Job drawing, mm, ordinate dimensions from the low corner. One solid piece. A direction names the side the tool comes from. Give positions to 0.01 mm unless a question says otherwise; leave off trailing zeros. Write each loop counter-clockwise with the first axis right and the second up, starting at its lowest first coordinate (ties: lowest second). Pieces come first, ordered by that corner, then holes. Notation, with made-up numbers: (36.25, 86) - (93.25, 86) arc R12 ccw to (93.25, 95) - close; hole circle Ø8 at (7.25, -2.75). An arc over 180 degrees is marked (long way). Answer as a JSON object with one key per item and string values.
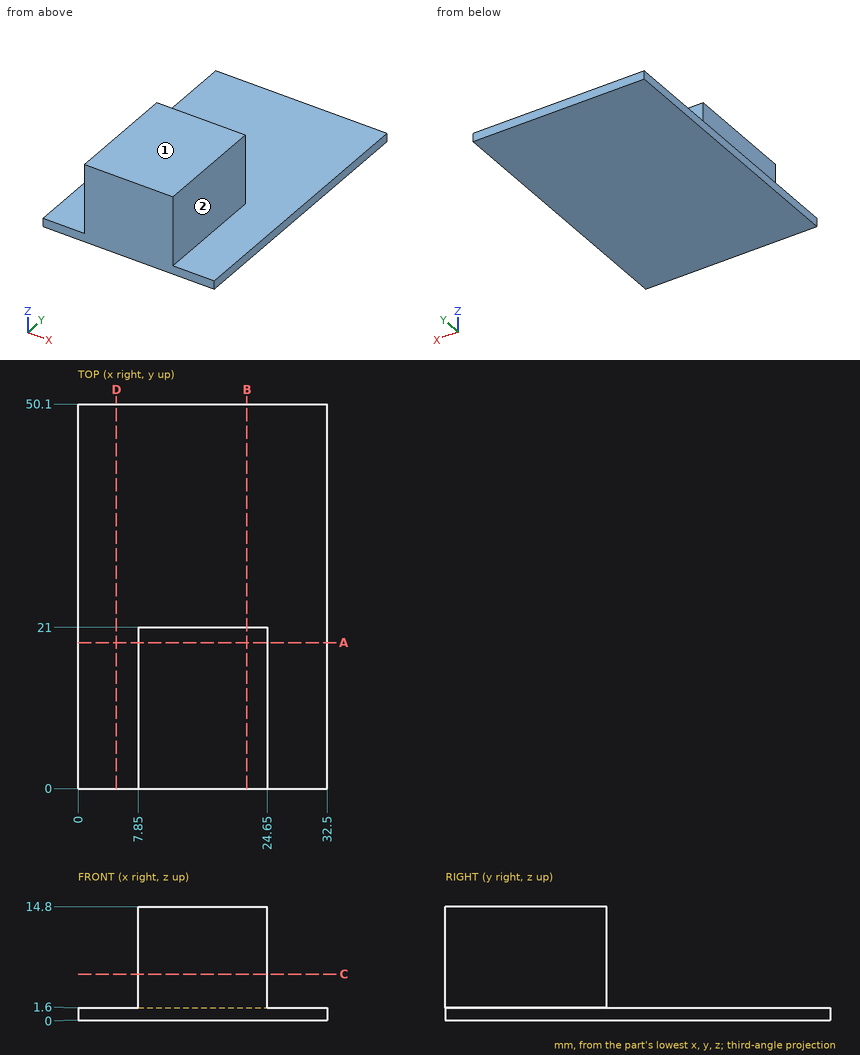
Item 1: Flat gauge pins, fed straight in: P1, Ø1.5, axis at x = 24, y = 30.5, coming from the +Z side; P2, Ø4, axis at x = 18.5, z = 6, coming from the +Y side; P3, Ø5, axis at y = 20.5, z = 13, coming from the -X side; P4, Ø1, axis at x = 26.5, y = 19, coming from the -Z side. Where does each tip first touch, or does it go through?
Entries:
{"P1": "z = 1.6", "P2": "y = 21", "P3": "x = 7.85", "P4": "z = 0"}
Item 2: Cut at C-C (z = 6). Give the cut face in (x, y).
Entries:
{"outline": "(7.85, 0) - (24.65, 0) - (24.65, 21) - (7.85, 21) - close"}
Item 3: Cut at D-D (x = 5). Give the cut face in (y, z), and give its area (3 significant figures).
Entries:
{"outline": "(0, 0) - (50.1, 0) - (50.1, 1.6) - (0, 1.6) - close", "area": "80.2 mm2"}
Item 4: Which spindle directions (+Z, -Z, +X, -X, +Y, -Y) get a long thin tool onto all of the face, cutting with end or side? Do the marked faces 1 and 2. Say none if no direction does.
Entries:
{"face 1": "+Z, +X, -X, +Y, -Y", "face 2": "+Z, +X, +Y, -Y"}
Item 5: Cut at B-B (x = 22). Give the cut face in (y, z), and give its area (3 significant figures).
Entries:
{"outline": "(0, 0) - (50.1, 0) - (50.1, 1.6) - (21, 1.6) - (21, 14.8) - (0, 14.8) - close", "area": "357 mm2"}
Item 6: Probe line 1 (X direction, y = 10.5, z = 11); line 2 (Z direction, x = 23, y = 40.5); line 3 (Y direction, x = 22, z = 12.75). List the from-to ranges inside material, lowest first. Write a range as from..to.
Entries:
{"line 1": "7.85..24.65", "line 2": "0..1.6", "line 3": "0..21"}
Item 7: Cut at A-A (y = 19). Give the cut face in (x, z).
Entries:
{"outline": "(0, 0) - (32.5, 0) - (32.5, 1.6) - (24.65, 1.6) - (24.65, 14.8) - (7.85, 14.8) - (7.85, 1.6) - (0, 1.6) - close"}
